CAD build for the part. Positions are in the model's coordinates, mm. Face numbers are marked on the shaded views. A direction names the side the tool comes from. Coordinates: 2 decimals unless noted, no trailing zeros. Write each loop counter-clockwise with the first axis right and the second up, starting at its lowest first coordinate (ties: lowest second). Pieces come first, ordered by that corner, then holes. Notation, with made-up numbers: M 1.5,12.25 L 39.5,12.25 A23 cw 39.5,36.25 Z; hole C 56,4 d3. An arc over 180 degrees is marked long. Answer as CSV lines item,"result". Start each with the question number.
Autodesk Inventor part; units mm, degrees
ref_plane "YZ Plane" through (0, 0, 0) normal (1, 0, 0) x (0, 1, 0)
ref_plane "XZ Plane" through (0, 0, 0) normal (0, 1, 0) x (-1, 0, 0)
ref_plane "XY Plane" through (0, 0, 0) normal (0, 0, 1) x (1, 0, 0)
sketch "Sketch1" plane through (0, 0, 0) normal (0, 1, 0) x (-1, 0, 0)
  line L0 (0, 0) -> (38.7, 0)
  line L1 (38.7, 0) -> (38.7, -44.5)
  line L2 (38.7, -44.5) -> (0, -44.5)
  line L3 (0, -44.5) -> (0, 0)
  line L4 (38.7, -22.25) -> (0, -22.25)
  line L5 (19.35, 0) -> (19.35, -44.5)
  dimension "d0" = 38.7
  dimension "d1" = 44.5
extrude "Extrusion1" add sketch "Sketch1" along normal blind 5
sketch "Sketch2" plane through (0, 5, 0) normal (0, 1, 0) x (1, 0, 0)
  circle A0 centre (-34.2, 4.5) radius 2
  line L0 (-38.7, 0) -> (0, 0)
  line L1 (-38.7, 44.5) -> (-38.7, 0)
  circle A1 centre (-34.2, 40) radius 2
  line L2 (0, 44.5) -> (-38.7, 44.5)
  circle A2 centre (-4.5, 4.5) radius 2
  line L3 (0, 0) -> (0, 44.5)
  circle A3 centre (-4.5, 40) radius 2
  dimension "d16" = 4
  dimension "d17" = 4.5
  dimension "d18" = 4.5
  dimension "d19" = 4
  dimension "d20" = 4.5
  dimension "d21" = 4.5
  dimension "d22" = 4
  dimension "d23" = 4.5
  dimension "d24" = 4.5
  dimension "d25" = 4
  dimension "d26" = 4.5
  dimension "d27" = 4.5
extrude "Extrusion2" add sketch "Sketch2" along normal blind 4 contours A0 | A1 | A2 | A3
sketch "Sketch3" plane through (-34.2, 9, -40) normal (0, 1, 0) x (1, 0, 0)
  circle A0 centre (0, 0) radius 1.35
  circle A1 centre (29.7, 0) radius 2
  circle A2 centre (29.7, 0) radius 1.35
  circle A3 centre (29.7, -35.5) radius 2
  circle A4 centre (29.7, -35.5) radius 1.35
  circle A5 centre (0, -35.5) radius 2
  circle A6 centre (0, -35.5) radius 1.35
  point P0 (34.2, -40)
  dimension "d30" = 2.7
  dimension "d31" = 2.7
  dimension "d32" = 2.7
  dimension "d33" = 2.7
extrude "Extrusion3" add sketch "Sketch3" along normal blind 4 contours A0 | A2 | A4 | A6
sketch "Sketch4" plane through (0, 0, 0) normal (0, -1, 0) x (1, 0, 0)
  circle A0 centre (-13, -6) radius 2.175
  line L0 (0, 0) -> (0, -44.5)
  line L1 (-38.7, 0) -> (0, 0)
  line L2 (-13, -6) -> (-13, -12)
  line L3 (-13, -12) -> (-7, -12)
  circle A1 centre (-7, -12) radius 2.175
  dimension "d36" = 4.35
  dimension "d37" = 13
  dimension "d38" = 6
  dimension "d39" = 6
  dimension "d40" = 6
  dimension "d41" = 4.35
hole "Hole1" at (-13, 0, -6) at (-7, 0, -12) direction (0, 1, 0) diameter 4.35 depth 4.5
properties part number "PCBMount"
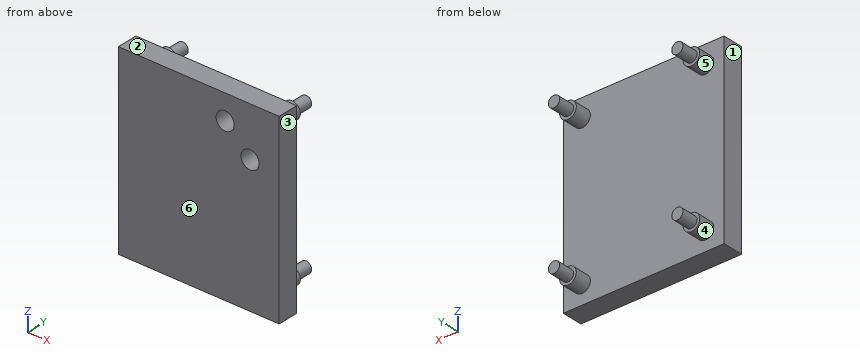
1) Band-saw the part on A-A, the plane z = -12. List the corners of the cut face in (x, y) (3 decimals), plus the area to 3 significant figures.
2) Probe L1, parallel to X at y = 3, z = -12 (3 decimals); L2, parallel to Z at x = -7, y = 2 (3 decimals); L3, parallel to Z at x = -13, y = 3.05 (3 decimals). List the from-to ranges inside material, lowest first. Write a range as [from, to].
3) Tool access for the marked faces 5 and 6: list every direction of +Z, -Z, +X, -X, +Y, -Y with a clear straight run to the whole face (end or side of a thin tool).
4) Band-saw the part on B-B, the plane y = 2.25. List the corners of the cut face in (x, z) (3 decimals), plus the area to 3 significant figures.
5) Pin check, flat tips, straight feed: P1, Ø4, axis at x = -7, z = -12, coming from the +Y side; P2, Ø2, axis at x = -13.5, z = -5.5, coming from the -Y side. Stop position of each tip, or through.
6) Band-saw the part on C-C, the plane x = -34.2. List the corners of the cut face in (y, z), plus the area to 3 significant figures.
7) Band-saw the part on D-D, the plane z = -40. List the corners of the cut face in (x, y), plus the area to 3 significant figures.
8) Two-plate mould, pull along X, no slides. Class the marked faces 1, 2, 3 and 4: pulls with the +X half, pulls with the -X half, needs draft (parallel to the pull), parting line crosses it, or undercut.
Result sheet:
1,outline,"M -38.7,0 L -9.175,0 L -9.175,4.5 L -4.825,4.5 L -4.825,0 L 0,0 L 0,5 L -38.7,5 Z"
1,area,"174 mm²"
2,L1,"x = [-38.7, -9.175], [-4.825, 0]"
2,L2,"z = [-44.5, -14.175], [-9.825, 0]"
2,L3,"z = [-44.5, -8.175], [-3.825, 0]"
3,face 5,"+Y"
3,face 6,"+Z, -Z, +X, -X, -Y"
4,outline,"M -38.7,-44.5 L 0,-44.5 L 0,0 L -38.7,0 Z; hole C -13,-6 d4.35; hole C -7,-12 d4.35"
4,area,"1,690 mm²"
5,P1,"stops at y = 5"
5,P2,"stops at y = 4.5"
6,outline,"M 0,-44.5 L 5,-44.5 L 5,-42 L 9,-42 L 9,-41.35 L 13,-41.35 L 13,-38.65 L 9,-38.65 L 9,-38 L 5,-38 L 5,-6.5 L 9,-6.5 L 9,-5.85 L 13,-5.85 L 13,-3.15 L 9,-3.15 L 9,-2.5 L 5,-2.5 L 5,0 L 0,0 Z"
6,area,"276 mm²"
7,outline,"M -38.7,0 L 0,0 L 0,5 L -2.5,5 L -2.5,9 L -3.15,9 L -3.15,13 L -5.85,13 L -5.85,9 L -6.5,9 L -6.5,5 L -32.2,5 L -32.2,9 L -32.85,9 L -32.85,13 L -35.55,13 L -35.55,9 L -36.2,9 L -36.2,5 L -38.7,5 Z"
7,area,"247 mm²"
8,face 1,"pulls with the -X half"
8,face 2,"needs draft"
8,face 3,"pulls with the +X half"
8,face 4,"undercut"
